Input: part model. Units: mm. Frame: model coordinates. A direction names the side the tool comes from. Coordinates: 2 decimals unless noted, no trailing zeros. Write each loop counter-clockwise with the first axis right and the second up, starting at its lowest first coordinate (ties: lowest second). Pieces come first, ordered by that corner, then holes.
1) Section query C-C (y = 54). Output: boundary loops of the cut face in (x, z), then the cut area to 3 significant figures.
2) Section query B-B (z = 13). Output: boundary loops of the cut face in (x, y), then the cut area to 3 significant figures.
3) Line query: L1, parallel to Y at x = 564.7, z = -0.5; L2, parallel to Z at x = 254, y = 49.5; L3, parallel to Y at x = 107, z = 6.75. Output: solid intervals per line, ascending.
4) Section query A-A (x = 114.5). Output: boundary loops of the cut face in (y, z), then the cut area to 3 significant figures.
5) Pin query (flat end, axial travel): pin 1 Ø4 at (x, y) = (363, 54) entering from +Z; pin 2 Ø12 at (x, z) = (482.5, 12.5) entering from -Y; pin 3 Ø12 at (y, z) = (66, 5.5) entering from +X. Return the tip coordinate at first contact, or that it passes through.
6) Set-up query: faces 1 (the flat face through (294, 91, 13)), 2 (the flat face through (294, 89.8, 13)). Return all of +Z, -Z, +X, -X, +Y, -Y with unobstructed straight access to the full face (end or side cutting, diameter ignored); none if empty.
from build123d import *

# Parameters (mm, degrees)
SKETCH1_W                    = 580
SKETCH1_H                    = 91
BASE_FLANGE1_DEPTH           = 1.2
EDGE_FLANGE2_STRIP_W         = 8.8
EDGE_FLANGE2_STRIP_H         = 1.2
EDGE_FLANGE2_STRIP_CUT_DEPTH = 580
EDGE_FLANGE2_DEPTH           = 580
CUT_EXTRUDE1_START           = -1.2
CUT_EXTRUDE1_OUTLINE_R       = 2.5
CUT_EXTRUDE1_DEPTH           = 1.2
CUT_EXTRUDE2_DEPTH           = 811.392138245
CUT_EXTRUDE2_DEPTH_BACK      = 811.392138245
SKETCH18_R                   = 2.5


# Read off the part's stored shape, not the designer's step: Cut-Extrude1
# Sheet-metal steps are written as plain solids
with BuildPart() as part:
    # Sketch1 → Base-Flange1 (new body)
    with BuildSketch(Plane.XY):
        with Locations((290, 45.5)):
            Rectangle(SKETCH1_W, SKETCH1_H)
    extrude(amount=-BASE_FLANGE1_DEPTH)

    # Edge-Flange2 strip (across the edge) → Edge-Flange2 strip cut (cut)
    with BuildSketch(Plane(origin=(580, 91, 0), x_dir=(0, -1, 0), z_dir=(-1, 0, 0))):
        with Locations((-1.2, -0.6)):
            Rectangle(EDGE_FLANGE2_STRIP_W, EDGE_FLANGE2_STRIP_H)
    extrude(amount=EDGE_FLANGE2_STRIP_CUT_DEPTH, mode=Mode.SUBTRACT)

    # Edge-Flange2 section (across the edge) → Edge-Flange2 (add)
    with BuildSketch(Plane(origin=(580, 91, 0), x_dir=(0, -1, 0), z_dir=(-1, 0, 0))):
        with BuildLine():
            Line((0, 2), (0, 23.8))
            Line((0, 23.8), (1.2, 23.8))
            Line((1.2, 23.8), (1.2, 2))
            ThreePointArc((1.2, 2), (1.785786438, 0.585786438), (3.2, 0))
            Line((3.2, 0), (3.2, -1.2))
            ThreePointArc((3.2, -1.2), (0.9372583, -0.2627417), (0, 2))
        make_face()
    extrude(amount=EDGE_FLANGE2_DEPTH)

    # Cut-Extrude1 outline → Cut-Extrude1 (cut)
    with BuildSketch(Plane.XY.offset(CUT_EXTRUDE1_START)):
        with Locations((15.3, 32.2)):
            Circle(CUT_EXTRUDE1_OUTLINE_R)
    extrude(amount=CUT_EXTRUDE1_DEPTH, mode=Mode.SUBTRACT)

    # Sketch18 → Cut-Extrude2 (cut, two sides: drawn at the far end of the back side and taken through both)
    with BuildSketch(Plane.XY.offset(-534.818311308).offset(-CUT_EXTRUDE2_DEPTH_BACK)):
        with Locations(Location((15.3, 32.2, 0), (0, 0, 180))):
            Circle(SKETCH18_R)
        with Locations(Location((564.7, 32.2, 0), (0, 0, 180))):
            Circle(SKETCH18_R)
    extrude(amount=CUT_EXTRUDE2_DEPTH + CUT_EXTRUDE2_DEPTH_BACK, mode=Mode.SUBTRACT)


solid = part.part
Answer:
1. outline: (0, -1.2) - (580, -1.2) - (580, 0) - (0, 0) - close
1. area: 696 mm2
2. outline: (0, 89.8) - (580, 89.8) - (580, 91) - (0, 91) - close
2. area: 696 mm2
3. L1: y = 0 to 29.7, 34.7 to 89.8
3. L2: z = -1.2 to 0
3. L3: y = 89.8 to 91
4. outline: (0, -1.2) - (87.8, -1.2) arc R3.2 ccw to (91, 2) - (91, 23.8) - (89.8, 23.8) - (89.8, 2) arc R2 cw to (87.8, 0) - (0, 0) - close
4. area: 136 mm2
5. pin 1: stops at z = 0
5. pin 2: stops at y = 89.8
5. pin 3: stops at x = 580
6. face 1: +Z, -Z, +X, -X, +Y
6. face 2: +Z, +X, -X, -Y
